Autodesk Inventor part; units mm, degrees
ref_plane "YZ Plane" through (0, 0, 0) normal (1, 0, 0) x (0, 1, 0)
ref_plane "XZ Plane" through (0, 0, 0) normal (0, 1, 0) x (-1, 0, 0)
ref_plane "XY Plane" through (0, 0, 0) normal (0, 0, 1) x (1, 0, 0)
sketch "Sketch1" plane through (0, 0, 0) normal (0, 0, 1) x (1, 0, 0)
  line L0 (4.1808, 5.4587) -> (6.8178, 0.8913)
  line L1 (6.8178, -0.8913) -> (4.1808, -5.4587)
  line L2 (2.637, -6.35) -> (-2.637, -6.35)
  line L3 (-4.1808, -5.4587) -> (-6.8178, -0.8913)
  line L4 (-6.8178, 0.8913) -> (-4.1808, 5.4587)
  line L5 (-2.637, 6.35) -> (2.637, 6.35)
  arc A0 (-6.8178, 0.8913) -> (-6.8178, -0.8913) centre (0, 0) ccw
  arc A1 (-4.1808, -5.4587) -> (-2.637, -6.35) centre (0, 0) ccw
  arc A2 (2.637, -6.35) -> (4.1808, -5.4587) centre (0, 0) ccw
  arc A3 (6.8178, -0.8913) -> (6.8178, 0.8913) centre (0, 0) ccw
  arc A4 (4.1808, 5.4587) -> (2.637, 6.35) centre (0, 0) ccw
  arc A5 (-2.637, 6.35) -> (-4.1808, 5.4587) centre (0, 0) ccw
  circle A6 centre (0, 0) radius 2.5527
  dimension "d2" = 12.7
  dimension "d3" = 6.8758
  dimension "d4" = 5.1054
extrude "Extrusion1" add sketch "Sketch1" along normal blind 101.6
properties part number "THUNDER HEX - 4" material "Aluminum 6061"
Design review of the part built by this model. Coordinates are the model's own, in mm. Round coordinates to 2 decimals unless told otherwise and drop trailing zeros. Write each loop counter-clockwise with the first axis right and the second up, starting at its lowest first coordinate (ties: lowest second). Pieces come first, ordered by that corner, then holes. Notation, with made-up numbers: (18.25, 52) -> (38.25, 52) arc R21 ccw to (38.25, 90) -> close; hole circle Ø2 at (-30.75, 83). An arc over 180 degrees is marked (long way). Answer in a Markdown table with one row per item.
Q1. Take a section at C-C, the plane x = 0. State the section outline as (y, z) points.
The answers:
| item | result |
|---|---|
| outline | (-6.35, 0) -> (-2.55, 0) -> (-2.55, 101.6) -> (-6.35, 101.6) -> close; (2.55, 0) -> (6.35, 0) -> (6.35, 101.6) -> (2.55, 101.6) -> close |
Q2. To check wall thickness, follow L1, parallel to Y at x = 0, z = 78; L2, parallel to Y at x = -0.25, z = 46; L3, parallel to X at y = -1.25, z = 39.5. State the ranges of each line that lie inside material, in increasing order. Write a range as [from, to].
The answers:
| item | result |
|---|---|
| L1 | [-6.35, -2.55], [2.55, 6.35] |
| L2 | [-6.35, -2.54], [2.54, 6.35] |
| L3 | [-6.61, -2.23], [2.23, 6.61] |
Q3. Take a section at B-B, the plane y = 0. State the section outline as (x, z) points, then the cut area to 3 significant figures.
The answers:
| item | result |
|---|---|
| outline | (-6.88, 0) -> (-2.55, 0) -> (-2.55, 101.6) -> (-6.88, 101.6) -> close; (2.55, 0) -> (6.88, 0) -> (6.88, 101.6) -> (2.55, 101.6) -> close |
| area | 878 mm² |
Q4. Take a section at A-A, the plane z = 29. State the section outline as (x, y) points.
The answers:
| item | result |
|---|---|
| outline | (-6.82, -0.89) -> (-4.18, -5.46) arc R6.87 ccw to (-2.64, -6.35) -> (2.64, -6.35) arc R6.88 ccw to (4.18, -5.46) -> (6.82, -0.89) arc R6.88 ccw to (6.82, 0.89) -> (4.18, 5.46) arc R6.87 ccw to (2.64, 6.35) -> (-2.64, 6.35) arc R6.88 ccw to (-4.18, 5.46) -> (-6.82, 0.89) arc R6.88 ccw to start; hole circle Ø5.11 at (0, 0) |
Q5. Clearance check with flat-ended pins moving along their axes: pin 1 Ø3 at (y, z) = (3, 62.5) entering from -X; pin 2 Ø3 at (x, y) = (2.5, 0) entering from +Z; pin 3 Ø1.5 at (y, z) = (2.5, 83.5) entering from +X. State where each tip first meets the part, or that it passes through.
The answers:
| item | result |
|---|---|
| pin 1 | x = -6.47 |
| pin 2 | z = 101.6 |
| pin 3 | x = 6.32 |
Q6. Take a section at D-D, the plane x = 5.5. State the section outline as (y, z) points.
The answers:
| item | result |
|---|---|
| outline | (-3.17, 0) -> (3.17, 0) -> (3.17, 101.6) -> (-3.17, 101.6) -> close |
